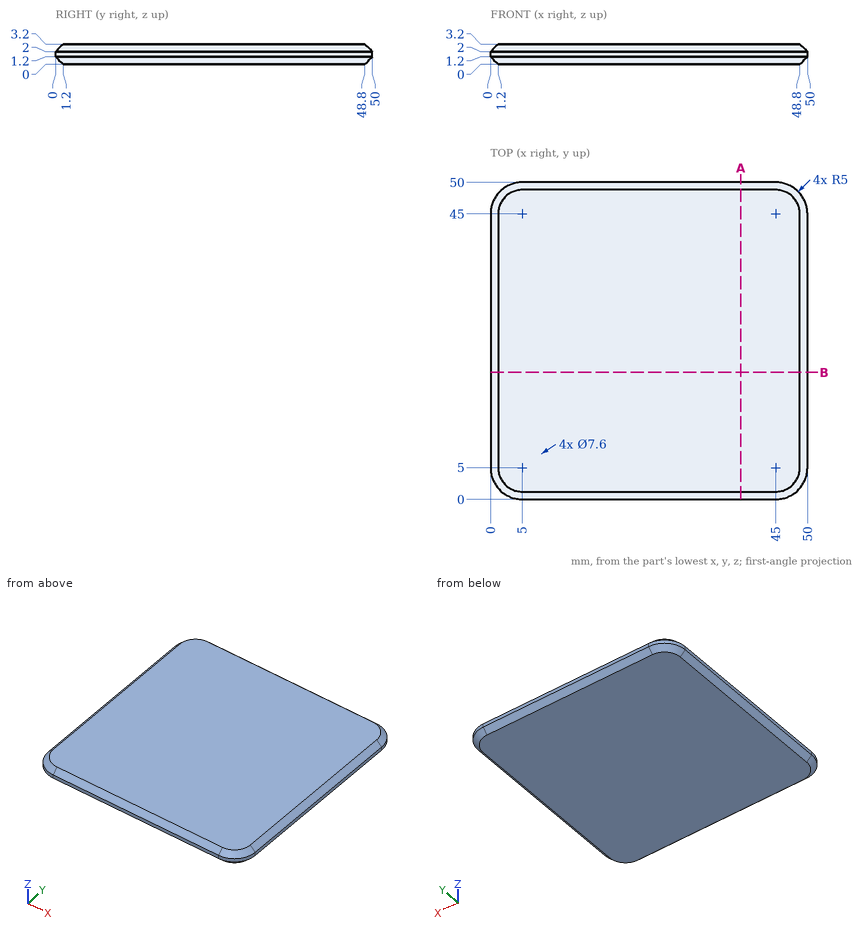
The figure shows three views and two pictorial views of one solid part (mm, origin at its lowest corner). Answer the questions. Coordinates: 2 decimals unless noted, no trailing zeros. Loops run counter-clockwise (first coordinate to the right, second up) from the corner with the lowest first, then second, coordinate; pieces in that order, holes last. Notation, with made-up numbers: (79.5, 48) - (136.5, 48) arc R12 cw to (136.5, 52) - close; hole circle Ø8 at (15, 17.25). An arc over 180 degrees is marked (long way). Answer in a Markdown table with one row per item.
Q1. Straight lines are drawn through the part: line 1 along X through (y, z) = (36, 0.9); line 2 along Y through (x, z) = (46.5, 1.75); line 3 along Y through (x, z) = (41, 0.4). For each, find the intervals that lie inside material, in ascending order. Write a range as [from, to].
Here are the results:
| item | result |
|---|---|
| line 1 | x = [0.3, 49.7] |
| line 2 | y = [0.23, 49.77] |
| line 3 | y = [0.8, 49.2] |
Q2. Find section A-A on x = 39.5. Write down the section's boundary in (y, z).
Here are the results:
| item | result |
|---|---|
| outline | (0, 1.2) - (1.2, 0) - (48.8, 0) - (50, 1.2) - (50, 2) - (48.8, 3.2) - (1.2, 3.2) - (0, 2) - close |
